Verification items for this drawing (mm, ordinates from the low corner). Give positions to 0.01 mm unless a question says otherwise; leave off trailing zeros. Write each loop counter-clockwise with the first axis right and the second up, starting at its lowest first coordinate (ties: lowest second). Pieces come first, ordered by that corner, then holes. Notation, with made-up numbers: (1.5, -25.75) -> (8.5, -25.75) arc R15 cw to (8.5, -16.75) -> close; hole circle Ø6 at (61.5, 57.25). An arc over 180 degrees is marked (long way). Answer as a JSON object with one key per item and string values.
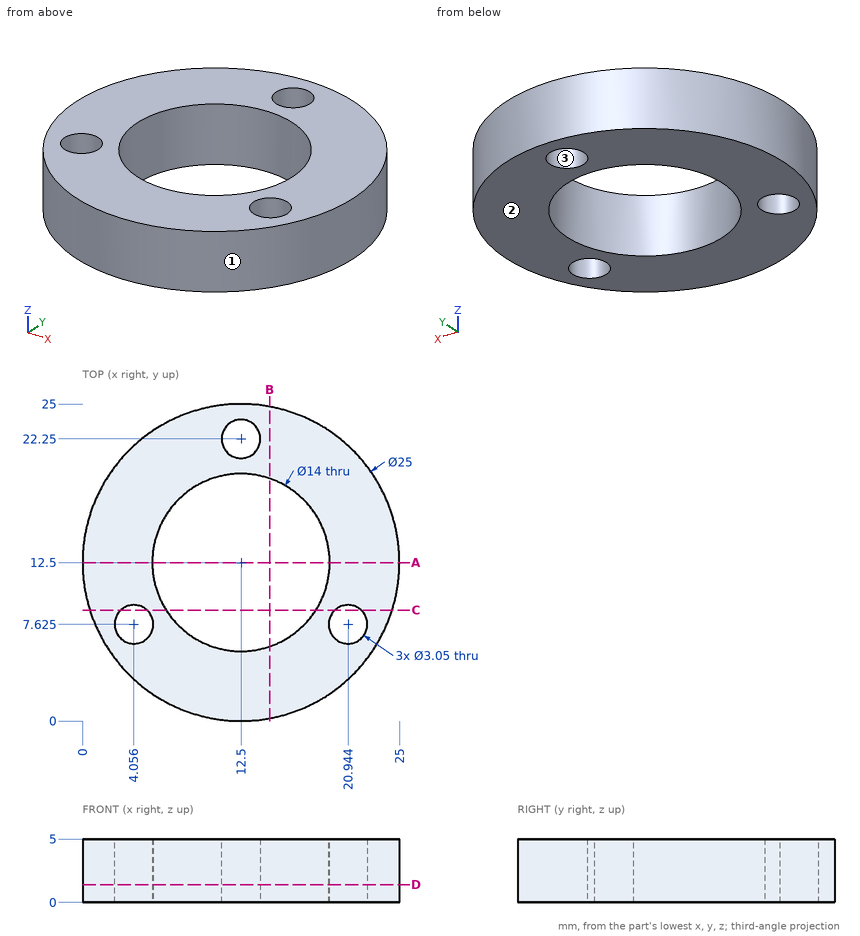
1. Sectioned sample at C-C, the plane y = 8.75. Enter the section's corners in (x, z).
Determined:
{"outline": "(0.58, 0) -> (3.03, 0) -> (3.03, 5) -> (0.58, 5) -> close; (5.09, 0) -> (6.59, 0) -> (6.59, 5) -> (5.09, 5) -> close; (18.41, 0) -> (19.91, 0) -> (19.91, 5) -> (18.41, 5) -> close; (21.97, 0) -> (24.42, 0) -> (24.42, 5) -> (21.97, 5) -> close"}
2. Go/stop test with flat-tipped pins: P1, Ø1, axis at x = 11.5, z = 1, coming from the -Y side; P2, Ø2.5, axis at x = 4.06, y = 7.62, coming from the +Z side; P3, Ø1, axis at y = 5.5, z = 3.5, coming from the +X side. Record where each tip stops, or that it passes through.
Determined:
{"P1": "y = 0.01", "P2": "through", "P3": "x = 23.18"}
3. Sectioned sample at A-A, the plane y = 12.5. Enter the section's corners in (x, z), plus the area to 3 significant figures.
Determined:
{"outline": "(0, 0) -> (5.5, 0) -> (5.5, 5) -> (0, 5) -> close; (19.5, 0) -> (25, 0) -> (25, 5) -> (19.5, 5) -> close", "area": "55.0 mm^2"}
4. Sectioned sample at B-B, the plane x = 14.75. Enter the section's corners in (y, z), plus the area to 3 significant figures.
Determined:
{"outline": "(0.2, 0) -> (5.87, 0) -> (5.87, 5) -> (0.2, 5) -> close; (19.13, 0) -> (24.8, 0) -> (24.8, 5) -> (19.13, 5) -> close", "area": "56.7 mm^2"}
5. Sectioned sample at D-D, the plane z = 1.4. State how many separate pieces and enclosed holes the cut face has, plus the area to 3 significant figures.
Determined:
{"separate pieces": "1", "enclosed holes": "4", "area": "315 mm^2"}
6. Mould release check, pull along X, two halves, no side actions. Record for the marked faces 1, 2 and 3: released by +X, released by -X, zero draft, split by the parting line, or undercut.
Determined:
{"face 1": "split by the parting line", "face 2": "zero draft", "face 3": "undercut"}
7. Scan lines: L1, parallel to Y at x = 12.5, z = 2.65 (1 decimal); L2, parallel to X at y = 7.5, z = 3.85 (1 decimal); L3, parallel to X at y = 10.25, z = 4.35 (1 decimal). Record each from-to range of solid material in increasing order. Write a range as [from, to].
Determined:
{"L1": "[0, 5.5], [19.5, 20.7], [23.8, 25]", "L2": "[1, 2.5], [5.6, 7.6], [17.4, 19.4], [22.5, 24]", "L3": "[0.2, 5.9], [19.1, 24.8]"}
